```python
from build123d import *

# Parameters (mm, degrees)
CIRCUNFERENCES_R     = 20
CIRCUNFERENCES_R_2   = 13.15
EXT_DEPTH            = 3
CIRCUNFERENCES_3_R   = 13.15
CIRCUNFERENCES_3_R_2 = 11.15
CENT_DEPTH           = 30
ARM_START            = -3
ARMS_R               = 1.65
ARM_DEPTH            = 3
CIRPATTERN1_COUNT    = 4
CHAMFER1_SIZE        = 2
CHAMFER2_SIZE        = 2
FILLET1_R            = 2


with BuildPart() as part:
    # Circunferences → EXT (new body)
    with BuildSketch(Plane(origin=(0, 0, 0), x_dir=(1, 0, 0), z_dir=(0, 1, 0))):
        with Locations(Location((0, 0, 0), (0, 0, 270))):
            Circle(CIRCUNFERENCES_R)
        with Locations(Location((0, 0, 0), (0, 0, 270))):
            Circle(CIRCUNFERENCES_R_2, mode=Mode.SUBTRACT)
    extrude(amount=EXT_DEPTH)

    # Circunferences<3> → CENT (add)
    with BuildSketch(Plane(origin=(0, 0, 0), x_dir=(1, 0, 0), z_dir=(0, 1, 0))):
        with Locations(Location((0, 0, 0), (0, 0, 270))):
            Circle(CIRCUNFERENCES_3_R)
        with Locations(Location((0, 0, 0), (0, 0, 270))):
            Circle(CIRCUNFERENCES_3_R_2, mode=Mode.SUBTRACT)
    extrude(amount=CENT_DEPTH)

    # ARMS → ARM (add)
    with BuildSketch(Plane(origin=(0, 3, 0), x_dir=(1, 0, 0), z_dir=(0, 1, 0)).offset(ARM_START)):
        with BuildLine():
            Line((25, 4), (19.595917942, 4))
            ThreePointArc((19.595917942, 4), (19.89872306, 2.01017924), (20, 0))
            ThreePointArc((20, 0), (19.89872306, -2.01017924), (19.595917942, -4))
            Line((19.595917942, -4), (25, -4))
            ThreePointArc((25, -4), (29, 0), (25, 4))
        make_face()
        with Locations(Location((25, 0, 0), (0, 0, 270))):
            Circle(ARMS_R, mode=Mode.SUBTRACT)
    arm = extrude(amount=ARM_DEPTH)

    # CirPattern1: ARM ×4 about axis
    cirpattern1_axis = Axis((0, 0, 0), (0, 1, 0))
    for i in range(1, CIRPATTERN1_COUNT):
        add(arm.rotate(cirpattern1_axis, i * 360 / CIRPATTERN1_COUNT))

    # Chamfer1
    chamfer1_edges = [part.edges().sort_by_distance(p)[0] for p in [
        (0, 0, -11.15),
    ]]
    chamfer(chamfer1_edges, length=CHAMFER1_SIZE)

    # Chamfer2
    chamfer2_edges = [part.edges().sort_by_distance(p)[0] for p in [
        (0, 3, -13.15),
    ]]
    chamfer(chamfer2_edges, length=CHAMFER2_SIZE)

    # Fillet1
    fillet1_edges = [part.edges().sort_by_distance(p)[0] for p in [
        (0, 30, -13.15),
    ]]
    fillet(fillet1_edges, radius=FILLET1_R - 0.0001)  # a hair under: the kernel refuses the full size


solid = part.part
```
The model under review builds one solid part; all positions refer to its coordinate system, in mm. A direction names the side the tool comes from. Round coordinates to 2 decimals unless told otherwise and drop trailing zeros. Order: outer loops, then holes, each group sorted by start corner. A loop starts at its lowest first (then second) coordinate and runs counter-clockwise, first axis right, second up.
Item 1: Add section D-D, the plane x = 22.5. State the section outline as (y, z) points.
Working result:
outline: (0, -4) - (3, -4) - (3, 4) - (0, 4) - close
Item 2: For pin 1 (1.5 mm diameter, centred on y = 1.5, z = 23, fed in from -X); pin 2 (2 mm diameter, centred on x = 0, z = -25, fed in from +Y); pin 3 (12 mm diameter, centred on x = 13.5, y = 23, fed in from -Z); pin 4 (3.5 mm diameter, centred on x = -21.5, y = 1, fed in from -Z), all flat-tipped, find the tip position at first contact; note any pin that passes through.
Working result:
pin 1: stops at x = -4
pin 2: passes through
pin 3: stops at z = -10.8
pin 4: stops at z = -4
Item 3: Draft analysis for pull direction Z (two halves, no side actions). For faces 5 (the cylindrical face through (26.636, 1.479, -0.215)), 6 (the cylindrical face through (29, 1, 0)), 7 (the flat face through (4, 1, 22)), state which applies: released by +Z, released by -Z, zero draft, split by the parting line, or undercut.
Working result:
face 5: undercut
face 6: split by the parting line
face 7: zero draft
Item 4: Machinability: for faces 1 (the flat face through (-22, 1, 4)), 2 (the flat face through (22, 1, 4)), 3 (the cylindrical face through (-5.037, 16.339, 12.147)), 4 (the flat face through (-22, 1, -4)), which of the approach directions +Z, -Z, +X, -X, +Y, -Y give a long, thin tool a straight path to every point of the face, cutting with its end or side? Answer none if there is none.
Working result:
face 1: +Z, -X, +Y, -Y
face 2: +Z, +X, +Y, -Y
face 3: +Y
face 4: -Z, -X, +Y, -Y
Item 5: Add section C-C, the plane y = 15. State the section outline as (x, z) points, and give its area (3 significant figures).
Working result:
outline: circle Ø26.3 at (0, 0); hole circle Ø22.3 at (0, 0)
area: 153 mm2
Item 6: To check wall thickness, follow probe 1 along X at (y, z) = (2.25, 0); probe 2 along X at (y, z) = (1.5, -25); probe 3 along X at (y, z) = (20.75, 0). State the ranges of each line that lie inside material, in increasing order.
Working result:
probe 1: x = -29 to -26.65, -23.35 to -11.15, 11.15 to 23.35, 26.65 to 29
probe 2: x = -4 to -1.65, 1.65 to 4
probe 3: x = -13.15 to -11.15, 11.15 to 13.15
Item 7: Add section A-A, the plane x = 0. Count the separate pieces of the cut face and the enclosed holes in it, and give its area (3 significant figures).
Working result:
separate pieces: 4
enclosed holes: 0
area: 194 mm2
